Can you work these out from the model? Positions are in its coordinate system, mm. Face numbers are marked on the shaded views. Round coordinates to 2 decimals unless told otherwise and drop trailing zeros. Order: outer loops, then holes, each group sorted by start corner. A loop starts at its lowest first (then second) coordinate and runs counter-clockwise, first axis right, second up.
Q1. If we section it at A-A (x = 70): Please give me the cut outline in (y, z), plus the area to 3 significant figures.
Q2. We'd pull the mould along X, two halves only. Please class the marked faces 1 and 2: pulls with the +X half, pulls with the -X half, needs draft (parallel to the pull), parting line crosses it, or undercut.
Q3. Will these pins go through, and if not, where does the flat tip stop? P1, Ø1.2, axis at x = -17.5, y = -7, coming from the +Z side; P2, Ø5, axis at x = 41.5, y = -7, coming from the +Z side.
Q4. If I drill on line 1 (X direction, y = -7.25, z = 2.4); line 2 (Y direction, x = 70, z = 1.9); line 3 (Y direction, x = 58, z = 3.2), over which ranges is the centre line in solid material (lowest first)?
Q5. If we section it at B-B (x = 52): Please give me the cut outline in (y, z).
from build123d import *

# Parameters (mm, degrees)
F0_R          = 1
F0_R_2        = 1.5
F0_R_3        = 2
F0_R_4        = 2.5
F0_W          = 20
F0_H          = 13
F1_DEPTH      = 5
F2_DEPTH      = 5
F4_DEPTH      = 25
F6_DEPTH      = 25
F6_DEPTH_BACK = 25
F7_W          = 10
F7_H          = 13
F8_DEPTH      = 1
F9_W          = 10
F9_H          = 4
F10_DEPTH     = 1
F11_W         = 10
F11_H         = 4
F12_DEPTH     = 1


with BuildPart() as f1:
    # F0 (on Top) → F1 (new body)
    with BuildSketch(Plane.XY):
        with BuildLine():
            Line((51, 0), (0, 0))
            Line((0, 0), (0, -13))
            Line((0, -13), (80, -13))
            Line((80, -13), (80, 0))
            Line((80, 0), (72.5, 0))
            ThreePointArc((72.5, 0), (70, -2.5), (67.5, 0))
            Line((67.5, 0), (66, 0))
            ThreePointArc((66, 0), (64, -2), (62, 0))
            Line((62, 0), (59.5, 0))
            ThreePointArc((59.5, 0), (58, -1.5), (56.5, 0))
            Line((56.5, 0), (53, 0))
            ThreePointArc((53, 0), (52, -1), (51, 0))
        make_face()
        with Locations((52, -6.5)):
            Circle(F0_R, mode=Mode.SUBTRACT)
        with Locations((58, -6.5)):
            Circle(F0_R_2, mode=Mode.SUBTRACT)
        with Locations((64, -6.5)):
            Circle(F0_R_3, mode=Mode.SUBTRACT)
        with Locations((70, -6.5)):
            Circle(F0_R_4, mode=Mode.SUBTRACT)
        with Locations((-10, -6.5)):
            Rectangle(F0_W, F0_H)
    extrude(amount=F1_DEPTH)

    # F0 (on Top) → F2 (join)
    with BuildSketch(Plane.XY):
        with BuildLine():
            Line((80, 0), (80, -13))
            Line((80, -13), (100, -13))
            Line((100, -13), (100, -11.5))
            ThreePointArc((100, -11.5), (95, -6.5), (100, -1.5))
            Line((100, -1.5), (100, 0))
            Line((100, 0), (80, 0))
        make_face()
    extrude(amount=F2_DEPTH)

    # F3 (on face) → F4 (cut)
    with BuildSketch(Plane.XZ.offset(13)):
        with BuildLine():
            add(Edge.make_bspline(
                [(100, 5), (101.2132067544, 5.5826393103), (101.9557552568, 6.3039713147), (102.6983037591, 7.0253033191)],
                knots=[0.7752257758, 0.7752257758, 0.7752257758, 0.7752257758, 1, 1, 1, 1], degree=3))
            Line((100, 5), (100, 4))
            add(Edge.make_bspline(
                [(100, 4), (100.9116064462, 4.9781336211), (101.8049551027, 6.0017184701), (102.6983037591, 7.0253033191)],
                knots=[0.7146792603, 0.7146792603, 0.7146792603, 0.7146792603, 1, 1, 1, 1], degree=3))
        make_face()
        Polygon((0, 4), (0, 5), (-20, 5), (-20, 1), (-15, 1), (-15, 2), (-10, 2), (-10, 3), (-5, 3), (-5, 4), align=None)
        with BuildLine():
            Line((100, 5), (80, 5))
            add(Edge.make_bspline(
                [(80, 5), (84.0150963882, 4.2328291772), (91.3720317074, 2.8271278998), (98.0993371218, 4.0872117184), (100, 5)],
                knots=[0, 0, 0, 0, 0.4230846239, 0.7752257758, 0.7752257758, 0.7752257758, 0.7752257758], degree=3))
        make_face()
        with BuildLine():
            Line((100, 0), (100, 4))
            add(Edge.make_bspline(
                [(87.8586545587, 0), (91.1531912492, 0.2461096824), (96.7341711942, 0.6630220834), (99.0645185264, 2.9962490008), (100, 4)],
                knots=[0, 0, 0, 0, 0.4218859534, 0.7146792603, 0.7146792603, 0.7146792603, 0.7146792603], degree=3))
            Line((87.8586545587, 0), (100, 0))
        make_face()
    extrude(amount=-F4_DEPTH, mode=Mode.SUBTRACT)

    # F5 (on face) → F6 (cut, two sides)
    with BuildSketch(Plane.XY.offset(1)) as f6_sk:
        Polygon((8.119047619, -0.395), (10, 0), (10, 3.0941735022), (-21.7320173979, 3.0941735022), (-21.7320173979, -15.9472320229), (10, -15.9472320229), (10, -13), (8.119047619, -12.605), (8.119047619, -12.5), (7.619047619, -12.5), (5.7380952381, -12.105), (5.7380952381, -12), (5.2380952381, -12), (3.3571428571, -11.605), (3.3571428571, -11.5), (2.8571428571, -11.5), (0.9761904762, -11.105), (0.9761904762, -11), (0.4761904762, -11), (-1.4047619048, -10.605), (-1.4047619048, -10.5), (-1.9047619048, -10.5), (-3.7857142857, -10.105), (-3.7857142857, -10), (-4.2857142857, -10), (-6.1666666667, -9.605), (-6.1666666667, -9.5), (-6.6666666667, -9.5), (-8.5476190476, -9.105), (-8.5476190476, -9), (-9.0476190476, -9), (-10.9285714286, -8.605), (-10.9285714286, -8.5), (-11.4285714286, -8.5), (-13.3095238095, -8.105), (-13.3095238095, -8), (-13.8095238095, -8), (-15, -7.75), (-15, -13), (-20, -13), (-20, -6.75), (-20, -6.5), (-20, -6.25), (-20, 0), (-15, 0), (-15, -5.25), (-13.8095238095, -5), (-13.3095238095, -5), (-13.3095238095, -4.895), (-11.4285714286, -4.5), (-10.9285714286, -4.5), (-10.9285714286, -4.395), (-9.0476190476, -4), (-8.5476190476, -4), (-8.5476190476, -3.895), (-6.6666666667, -3.5), (-6.1666666667, -3.5), (-6.1666666667, -3.395), (-4.2857142857, -3), (-3.7857142857, -3), (-3.7857142857, -2.895), (-1.9047619048, -2.5), (-1.4047619048, -2.5), (-1.4047619048, -2.395), (0.4761904762, -2), (0.9761904762, -2), (0.9761904762, -1.895), (2.8571428571, -1.5), (3.3571428571, -1.5), (3.3571428571, -1.395), (5.2380952381, -1), (5.7380952381, -1), (5.7380952381, -0.895), (7.619047619, -0.5), (8.119047619, -0.5), align=None)
        Polygon((-15.6904761905, -5.395), (-15, -5.25), (-15, 0), (-20, 0), (-20, -6.25), (-18.5714285714, -6), (-18.0714285714, -6), (-18.0714285714, -5.895), (-16.1904761905, -5.5), (-15.6904761905, -5.5), align=None)
        Polygon((-15, -13), (-15, -7.75), (-15.6904761905, -7.605), (-15.6904761905, -7.5), (-16.1904761905, -7.5), (-18.0714285714, -7.105), (-18.0714285714, -7), (-18.5714285714, -7), (-20, -6.75), (-20, -13), align=None)
    extrude(amount=-F6_DEPTH, mode=Mode.SUBTRACT)
    extrude(f6_sk.sketch, amount=F6_DEPTH_BACK, mode=Mode.SUBTRACT)

    # F7 (on face) → F8 (cut)
    with BuildSketch(Plane.XY.offset(5)):
        with Locations((39.2707522213, -6.5)):
            Rectangle(F7_W, F7_H)
    extrude(amount=-F8_DEPTH, mode=Mode.SUBTRACT)

    # F9 (on face) → F10 (cut)
    with BuildSketch(Plane.XZ.offset(13)):
        with Locations((39.2707522213, 2)):
            Rectangle(F9_W, F9_H)
    extrude(amount=-F10_DEPTH, mode=Mode.SUBTRACT)

    # F11 (on face) → F12 (cut)
    with BuildSketch(Plane(origin=(0, 0, 0), x_dir=(-1, 0, 0), z_dir=(0, 1, 0))):
        with Locations((-39.2707522213, 2)):
            Rectangle(F11_W, F11_H)
    extrude(amount=-F12_DEPTH, mode=Mode.SUBTRACT)


solid = f1.part
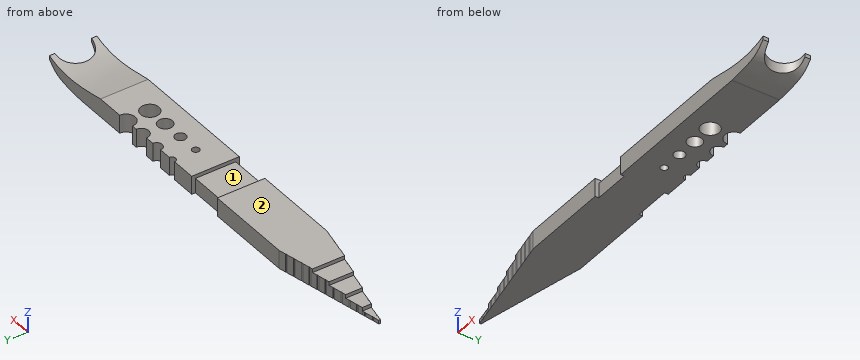
Solution:
1. outline: (-13, 0) - (-9, 0) - (-9, 5) - (-13, 5) - close; (-4, 0) - (-2.5, 0) - (-2.5, 5) - (-4, 5) - close
1. area: 27.5 mm2
2. face 1: undercut
2. face 2: needs draft
3. P1: stops at z = 1
3. P2: stops at z = 4
4. line 1: x = -10 to 51.34, 52.66 to 56.7, 59.3 to 62.15, 65.85 to 67.62, 72.38 to 95.06
4. line 2: y = -13 to -9, -4 to -2.5
4. line 3: y = -13 to -8, -5 to -1.5
5. outline: (-13, 0) - (-7.5, 0) - (-7.5, 5) - (-13, 5) - close; (-5.5, 0) - (-1, 0) - (-1, 5) - (-5.5, 5) - close
